The model under review builds one solid part; all positions refer to its coordinate system, in mm. A direction names the side the tool comes from. Give positions to 0.01 mm unless a question says otherwise; leave off trailing zeros. Write item = value, one per line. Start each with the question number.
1. We need section A-A, the plane x = 383. State how many separate pieces and enclosed holes the cut face has, and give its area (3 significant figures).
2. Wall thickness on probe 1 along Z at (x, y) = (354.5, -155.5); probe 2 along Z at (x, y) = (378, -254.5); probe 3 along X at (y, z) = (-131, -38): over which ranges is each line inside the solid? List them lowest first.
3. For P1, Ø4, axis at y = -107.5, z = 37, coming from the +X side; P2, Ø6, axis at y = -109.5, z = -3.5, coming from the -X side; P3, Ø12, axis at x = 328.63, y = -113.17, coming from the -Z side, all flat-tipped, find the tip position at first contact; note any pin that passes through.
4. Machinability: for faces 5 (the cylindrical face through (328.5, -113.4, -12)), 6 (the flat face through (312.92, -64.42, -9.83)), which of the approach directions +Z, -Z, +X, -X, +Y, -Y give a long, thin tool a straight path to every point of the face, cutting with its end or side? Answer none if there is none.
5. Mouldability with a two-part tool opening along Z and no side actions: class faces 1 (the cylindrical face through (328.8, -80.03, -0.53)), 2 (the flat face through (409.68, -317.71, 40.17)), 3 (the cylindrical face through (331.989, -122.587, 0.14)), 4 (the cylindrical face through (321.15, -106.53, 14.89)) as pulls with the +Z half, pulls with the -Z half, needs draft (parallel to the pull), parting line crosses it, or undercut.
from build123d import *

# Parameters (mm, degrees)
SWEEP_THIN1_PROFILE_R   = 12
SWEEP_THIN1_PROFILE_R_2 = 10


with BuildPart() as part:
    # Sweep-Thin1: sweep along a path in Sketch2
    with BuildLine(Plane(origin=(400, -300, 0), x_dir=(0, 0, -1), z_dir=(0.934155191329314, 0.35686703197758807, 0))) as sweep_thin1_path:
        Line((0, 251.145783), (0, 200))
        Line((0, 200), (-20, 200))
        ThreePointArc((-20, 200), (-41.213203, 191.213203), (-50, 170))
        Line((-50, 170), (-50, -20))
    # Sweep-Thin1 profile (on start of the path) → Sweep-Thin1 (sweep)
    with BuildSketch(Plane(origin=(310.37435, -65.390863, 0), x_dir=(-0.934155191329314, -0.35686703197758807, 0), z_dir=(0.35686703197758807, -0.934155191329314, 0))):
        Circle(SWEEP_THIN1_PROFILE_R)
        Circle(SWEEP_THIN1_PROFILE_R_2, mode=Mode.SUBTRACT)
    sweep_thin1 = sweep(path=sweep_thin1_path.line, transition=Transition.RIGHT)

    # Mirror1: Sweep-Thin1 across plane
    add(sweep_thin1.mirror(Plane.XY))


solid = part.part
Model answer:
q1.separate_pieces = 2
q1.enclosed_holes = 2
q1.area = 775 mm2
q2.probe_1 = -57.86 to -54.23, -45.77 to -42.14, 42.14 to 45.77, 54.23 to 57.86
q2.probe_2 = -61.2 to -59.02, -40.98 to -38.8, 38.8 to 40.98, 59.02 to 61.2
q2.probe_3 = 324.83 to 328.42, 338.69 to 342.35
q3.P1 = 339.33
q3.P2 = 313.56
q3.P3 = -54.47
q4.face_5 = none
q4.face_6 = +Z, -Z, -X, +Y
q5.face_1 = parting line crosses it
q5.face_2 = needs draft
q5.face_3 = undercut
q5.face_4 = undercut
